Verification items for the finished model (mm, model axes). Give positions to 0.01 mm unless a question says otherwise; leave off trailing zeros. Order: outer loops, then holes, each group sorted by start corner. A loop starts at its lowest first (then second) coordinate and runs counter-clockwise, first axis right, second up. Notation, with made-up numbers: (53.25, -0.5) -> (110.25, -0.5) arc R25 ccw to (110.25, 16.5) -> close; hole circle Ø6 at (-10, 4). An arc over 180 degrees is marked (long way). Return JSON: item names as keys, results as strings. Group by question number.
(1) Cross-section at B-B on x = -1.75. Enter the section's corners in (y, z), then the cut area to 3 significant figures.
(2) Cross-section at D-D on z = 0.9. State how many separate pieces and enclosed holes the cut face has, then the cut area to 3 significant figures.
(3) Cross-section at C-C on y = -27.5. Enter the section's corners in (x, z).
(4) Thickness scan on line 1 along Y through (x, z) = (-1.75, 1.7); line 2 along Y through (x, z) = (81.75, 2.95); line 3 along X through (y, z) = (-40.5, 3.05). Record the ranges inside material, lowest first.
(5) Cross-section at A-A on y = -38.8. Enter the section's corners in (x, z).
(6) Depth check by flat-ended pin: pin 1 Ø3 at (x, y) = (81.75, -38.8) entering from -Z; pin 2 Ø7 at (x, y) = (81.75, -27.5) entering from -Z. Enter the tip coordinate at first touch or a pass-through.
from build123d import *

# Parameters (mm, degrees)
ESQUISSE1_W             = 100
ESQUISSE1_H             = 50
BOSS_EXTRU_1_DEPTH      = 4
ESQUISSE2_R             = 1.5
ENL_V_MAT_EXTRU_1_DEPTH = 104.033974979
ESQUISSE3_R             = 4
ENL_V_MAT_EXTRU_2_DEPTH = 104.033974979
CONG_1_SIZE             = 3
ESQUISSE4_R             = 2.6
ESQUISSE4_R_2           = 2.49849628
ENL_V_MAT_EXTRU_3_DEPTH = 104.033974979


with BuildPart() as part:
    # Esquisse1 → Boss.-Extru.1 (new body)
    with BuildSketch(Plane.XY):
        with Locations((40, -25)):
            Rectangle(ESQUISSE1_W, ESQUISSE1_H)
    extrude(amount=BOSS_EXTRU_1_DEPTH)

    # Esquisse2 → Enlèv. mat.-Extru.1 (cut, through all)
    with BuildSketch(Plane(origin=(0, 0, 0), x_dir=(-1, 0, 0), z_dir=(0, 0, -1))):
        with Locations((-22.625, -7.625)):
            Circle(ESQUISSE2_R)
        with Locations((-57.375, -42.375)):
            Circle(ESQUISSE2_R)
        with Locations((-57.375, -7.625)):
            Circle(ESQUISSE2_R)
        with Locations((-22.5, -42.5)):
            Circle(ESQUISSE2_R)
    extrude(amount=-ENL_V_MAT_EXTRU_1_DEPTH, mode=Mode.SUBTRACT)

    # Esquisse3 → Enlèv. mat.-Extru.2 (cut, through all)
    with BuildSketch(Plane(origin=(0, 0, 0), x_dir=(-1, 0, 0), z_dir=(0, 0, -1))):
        with Locations((-39.984893454, -24.973718249)):
            Circle(ESQUISSE3_R)
    extrude(amount=-ENL_V_MAT_EXTRU_2_DEPTH, mode=Mode.SUBTRACT)

    # Congé1
    cong_1_edges = [part.edges().sort_by_distance(p)[0] for p in [
        (-10, 0, 2),
        (90, 0, 2),
        (90, -50, 2),
        (-10, -50, 2),
    ]]
    chamfer(cong_1_edges, length=CONG_1_SIZE)

    # Esquisse4 → Enlèv. mat.-Extru.3 (cut, through all)
    with BuildSketch(Plane.XY.offset(4)):
        with Locations((81.75, -27.5)):
            Circle(ESQUISSE4_R)
        with Locations((81.75, -38.8)):
            Circle(ESQUISSE4_R_2)
        with Locations((-1.75, -27.5)):
            Circle(ESQUISSE4_R)
        with Locations((-1.75, -38.8)):
            Circle(ESQUISSE4_R)
    extrude(amount=-ENL_V_MAT_EXTRU_3_DEPTH, mode=Mode.SUBTRACT)


solid = part.part
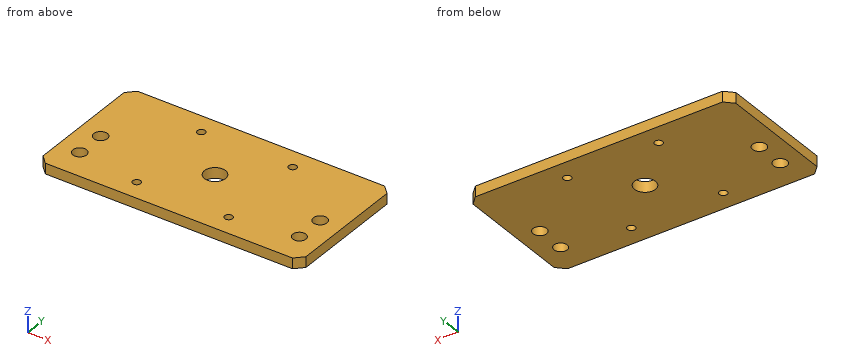
Verdict:
{
 "1": {"outline": "(-50, 0) -> (-41.4, 0) -> (-41.4, 4) -> (-50, 4) -> close; (-36.2, 0) -> (-30.1, 0) -> (-30.1, 4) -> (-36.2, 4) -> close; (-24.9, 0) -> (0, 0) -> (0, 4) -> (-24.9, 4) -> close", "area": "158 mm²"},
 "2": {"separate pieces": "1", "enclosed holes": "9", "area": "4,820 mm²"},
 "3": {"outline": "(-10, 0) -> (-4.35, 0) -> (-4.35, 4) -> (-10, 4) -> close; (0.85, 0) -> (36.88, 0) -> (36.88, 4) -> (0.85, 4) -> close; (43.09, 0) -> (79.15, 0) -> (79.15, 4) -> (43.09, 4) -> close; (84.35, 0) -> (90, 0) -> (90, 4) -> (84.35, 4) -> close"},
 "4": {"line 1": "-50 to -41.4, -36.2 to -30.1, -24.9 to 0", "line 2": "-50 to -41.3, -36.3 to -30.1, -24.9 to 0", "line 3": "-10 to -3.72, 0.22 to 79.92, 83.58 to 90"},
 "5": {"outline": "(-10, 0) -> (-4.35, 0) -> (-4.35, 4) -> (-10, 4) -> close; (0.85, 0) -> (79.25, 0) -> (79.25, 4) -> (0.85, 4) -> close; (84.25, 0) -> (90, 0) -> (90, 4) -> (84.25, 4) -> close"},
 "6": {"pin 1": "through", "pin 2": "z = 0"}
}
